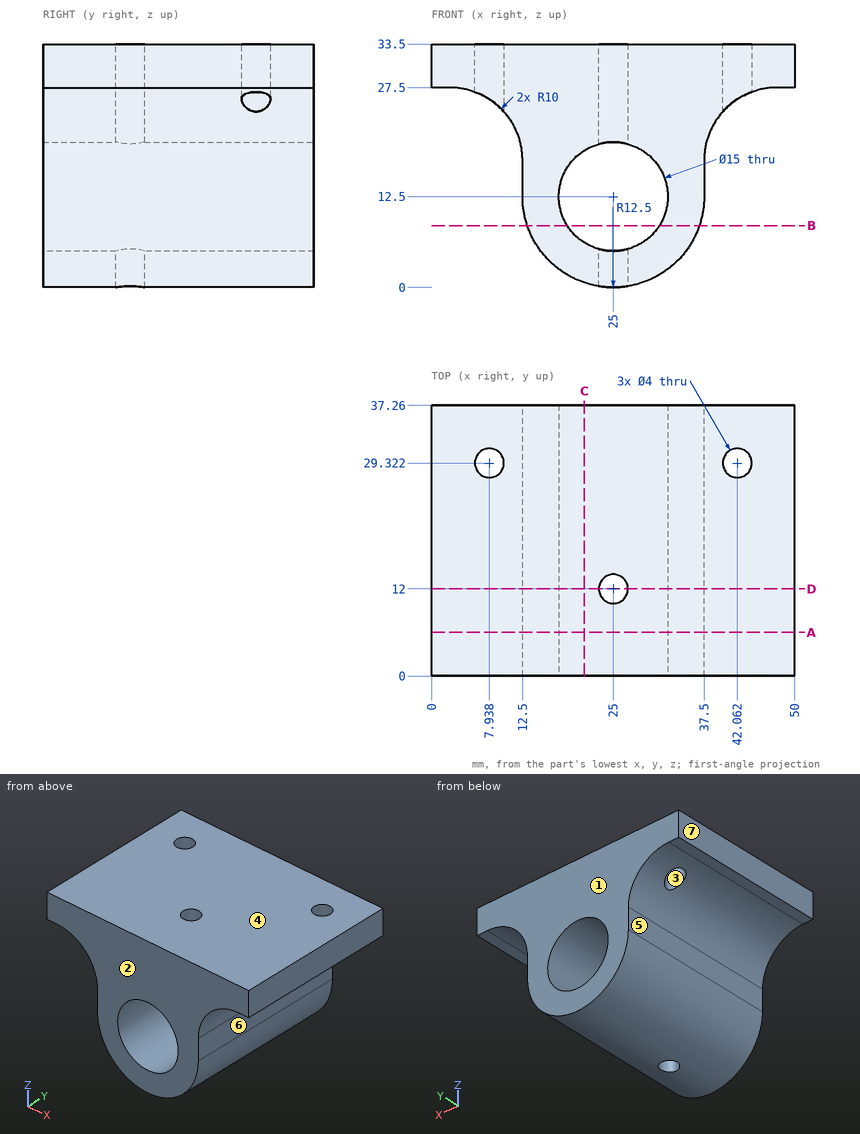
Study the drawing (mm; zero at the part's minimum x, y, z) and answer. A direction names the side the tool comes from. Coordinates: 2 decimals unless noted, no trailing zeros. Write each loop counter-clockwise with the first axis right and the second up, starting at its lowest first coordinate (ties: lowest second). Pieces come first, ordered by that corner, then holes.
Q1. Each of these flat-tipped pins is pushed along its axis until it touches: pin 1 Ø3 at (x, y) = (49.5, 25) entering from -Z; pin 2 Ø4 at (y, z) = (16, 14.5) entering from -X; pin 3 Ø2.5 at (y, z) = (11, 14.5) entering from +X. Where does it stop, or does it pass through?
Q2. A cutting plane is placed at D-D, the plane y = 12. Give the vertices of the cut face in (x, z).
Q3. Find the intervals of material crossed by line 1 (Y direction, x = 42, z = 30); line 2 (Z direction, x = 25, y = 27.5); line 3 (X direction, y = 19, z = 11), in increasing order.
Q4. Determine the mould class of the marked faces 1, 2, 3 and 4 for opening direction Y: released by +Y, released by -Y, zero draft, split by the parting line, or undercut.
Q5. A cutting plane is placed at C-C, the plane x = 21. Give the vertices of the cut face in (y, z) (1 decimal), then the cut area to 3 significant figures.
Q6. Which of the six approach directions +Z, -Z, +X, -X, +Y, -Y give full straight-line access (tool end or side, diameter ignored) to the marked faces 5, 6 and 7?
Q7. A cutting plane is placed at A-A, the plane y = 6. Give the vertices of the cut face in (x, z).
Q8. A cutting plane is placed at B-B, the plane z = 8.5. Give the vertices of the cut face in (x, y) (1 decimal).
Findings below:
1. pin 1: stops at z = 27.5
1. pin 2: stops at x = 12.5
1. pin 3: stops at x = 37.5
2. outline: (0, 27.5) - (2.5, 27.5) arc R10 cw to (12.5, 17.5) - (12.5, 12.5) arc R12.5 ccw to (23, 0.16) - (23, 5.27) arc R7.5 cw to (23, 19.73) - (23, 33.5) - (0, 33.5) - close; (27, 0.16) arc R12.5 ccw to (37.5, 12.5) - (37.5, 17.5) arc R10 cw to (47.5, 27.5) - (50, 27.5) - (50, 33.5) - (27, 33.5) - (27, 19.73) arc R7.5 cw to (27, 5.27) - close
3. line 1: y = 0 to 27.32, 31.32 to 37.26
3. line 2: z = 0 to 5, 20 to 33.5
3. line 3: x = 12.59 to 17.65, 32.35 to 37.41
4. face 1: released by +Y
4. face 2: released by -Y
4. face 3: undercut
4. face 4: zero draft
5. outline: (0, 0.7) - (37.3, 0.7) - (37.3, 6.2) - (0, 6.2) - close; (0, 18.8) - (37.3, 18.8) - (37.3, 33.5) - (0, 33.5) - close
5. area: 751 mm2
6. face 5: -Z, -X, +Y, -Y
6. face 6: -Z, +X, +Y, -Y
6. face 7: +Z, -Z, -X, +Y, -Y
7. outline: (0, 27.5) - (2.5, 27.5) arc R10 cw to (12.5, 17.5) - (12.5, 12.5) arc R12.5 ccw to (37.5, 12.5) - (37.5, 17.5) arc R10 cw to (47.5, 27.5) - (50, 27.5) - (50, 33.5) - (0, 33.5) - close; hole circle Ø15 at (25, 12.5)
8. outline: (13.2, 0) - (18.7, 0) - (18.7, 37.3) - (13.2, 37.3) - close; (31.3, 0) - (36.8, 0) - (36.8, 37.3) - (31.3, 37.3) - close
